Part print with two shaded views. Sizes in mm from the minimum x, y, z corner. Coordinates: 2 decimals unless noted, no trailing zeros. Write each loop counter-clockwise with the first axis right and the second up, starting at its lowest first coordinate (ties: lowest second). Pieces come first, ordered by that corner, then holes. Notation, with made-up numbers: (-36, 22.25) - (-10, 22.25) arc R26 cw to (-10, 38.25) - close; hole circle Ø4 at (-19, 3). An arc over 180 degrees is marked (long way). One line per question, with ' | ' between items. Start each with the question number.
1. Band-saw the part on A-A, the plane z = 2.7. Write the cut outline in (x, y).
2. Probe line 1 (Y direction, x = 25, z = 1); line 2 (Y direction, x = 24, z = 4.6); line 3 (X direction, y = 111.5, z = 1.7). List the from-to ranges inside material, lowest first.
3. Flat gauge pins, fed straight in: P1, Ø1, axis at y = 46, z = 3.5, coming from the -X side; P2, Ø1, axis at y = 84, z = 3, coming from the -X side. Where does each tip first touch, or does it go through?
4. Band-saw the part on C-C, the plane y = 10. Write the cut outline in (x, z), then the cut area to 3 significant figures.
5. Band-saw the part on B-B, the plane x = 25. Write the cut outline in (y, z).
6. Band-saw the part on D-D, the plane y = 82. Write the cut outline in (x, z).
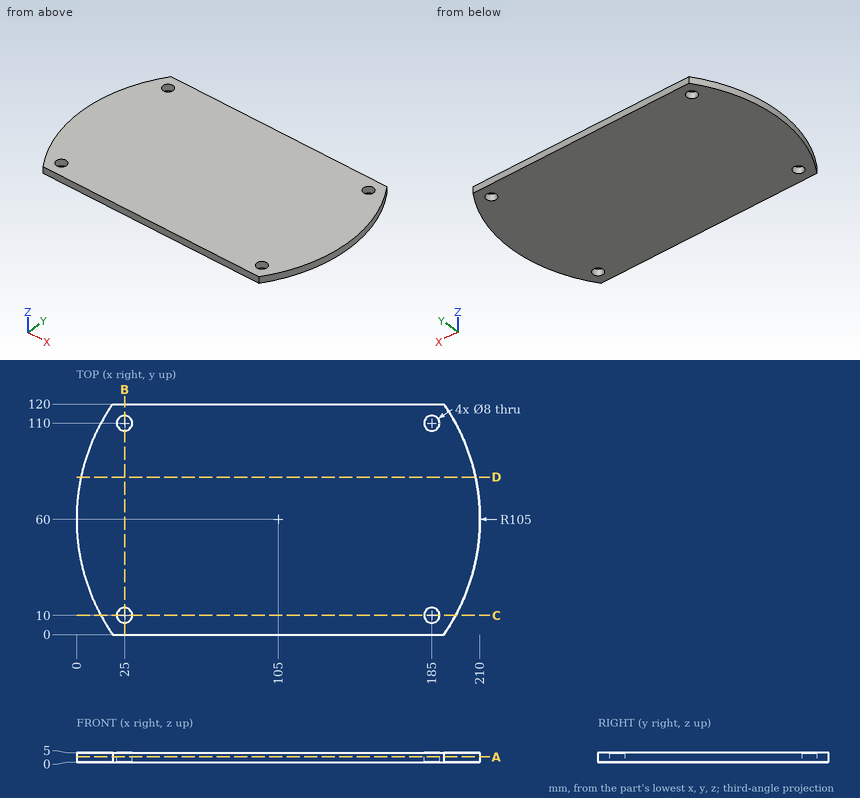
Filled in:
1) outline: (18.83, 0) - (191.17, 0) arc R105 ccw to (191.17, 120) - (18.83, 120) arc R105 ccw to start; hole circle Ø8 at (25, 10); hole circle Ø8 at (25, 110); hole circle Ø8 at (185, 10); hole circle Ø8 at (185, 110)
2) line 1: y = 0 to 6, 14 to 106, 114 to 120 | line 2: y = 0 to 6.13, 13.87 to 106.13, 113.87 to 120 | line 3: x = 13.5 to 21.29, 28.71 to 181.29, 188.71 to 196.5
3) P1: stops at x = 0.87 | P2: stops at x = 2.66
4) outline: (12.67, 0) - (21, 0) - (21, 5) - (12.67, 5) - close; (29, 0) - (181, 0) - (181, 5) - (29, 5) - close; (189, 0) - (197.33, 0) - (197.33, 5) - (189, 5) - close | area: 843 mm²
5) outline: (0, 0) - (6, 0) - (6, 5) - (0, 5) - close; (14, 0) - (106, 0) - (106, 5) - (14, 5) - close; (114, 0) - (120, 0) - (120, 5) - (114, 5) - close
6) outline: (2.33, 0) - (207.67, 0) - (207.67, 5) - (2.33, 5) - close
